Check sheet for the modelled part. Datum: model origin and axes. Units: mm. Face numbers are marked on the shaded views. A direction names the side the tool comes from. Coordinates: 2 decimals unless noted, no trailing zeros. Loops run counter-clockwise (first coordinate to the right, second up) from the corner with the lowest first, then second, coordinate; pieces in that order, holes last.
```python
from build123d import *

# Parameters (mm, degrees)
F1_DEPTH       = 100
F2_W           = 86.5
F2_H           = 50
F3_DEPTH       = 90
F4_W           = 30
F4_H           = 45
F4_W_2         = 14
F4_H_2         = 25
F5_DEPTH       = 60
F7_D           = 4
F7_CSINK_D     = 8.7
F7_CSINK_ANGLE = 90
F8_SIZE        = 2
F9_SIZE        = 3


with BuildPart() as f1:
    # F0 (on Right) → F1 (new body)
    with BuildSketch(Plane.YZ):
        Polygon((-60, 0), (0, 0), (0, 60), (-40, 60), (-40, 100), (-60, 100), align=None)
    extrude(amount=F1_DEPTH)

    # F2 (on face) → F3 (cut)
    with BuildSketch(Plane.XY.offset(100)):
        with Locations((50, -30)):
            Rectangle(F2_W, F2_H)
    extrude(amount=-F3_DEPTH, mode=Mode.SUBTRACT)

    # F4 (on face) → F5 (cut)
    with BuildSketch(Plane(origin=(0, 0, 0), x_dir=(1, 0, 0), z_dir=(0, 0, -1))):
        with Locations((34.25, 22.5)):
            Rectangle(F4_W, F4_H)
        with Locations((74.25, 22.5)):
            Rectangle(F4_W_2, F4_H_2)
    extrude(amount=-F5_DEPTH, mode=Mode.SUBTRACT)

    # F7 (through all)
    with Locations(Plane(origin=(0, -55, 0), x_dir=(-1, 0, 0), z_dir=(0, 1, 0))):
        with Locations((-78.25, 90), (-21.75, 90), (-34.25, 25)):
            CounterSinkHole(F7_D / 2, F7_CSINK_D / 2, counter_sink_angle=F7_CSINK_ANGLE)

    # F8
    f8_edges = [f1.edges().sort_by_distance(p)[0] for p in [
        (74.625, 0, 60),
        (100, 0, 30),
        (0, 0, 30),
        (19.25, 0, 30),
        (49.25, -25, 10),
        (34.25, -45, 10),
        (49.25, 0, 30),
        (100, -20, 60),
        (93.25, -22.5, 60),
        (6.75, -22.5, 60),
        (0, -20, 60),
        (9.625, 0, 60),
        (0, -40, 80),
        (6.75, -40, 80),
        (93.25, -40, 80),
        (100, -40, 80),
        (3.375, -40, 100),
        (0, -50, 100),
        (6.75, -47.5, 100),
        (93.25, -47.5, 100),
        (96.625, -40, 100),
        (100, -50, 100),
        (50, -55, 100),
        (19.25, -2.5, 60),
        (49.25, -2.5, 60),
        (19.25, -25, 10),
    ]]
    chamfer(f8_edges, length=F8_SIZE)

    # F9
    f9_edges = [f1.edges().sort_by_distance(p)[0] for p in [
        (67.25, -22.5, 10),
        (74.25, -10, 10),
        (81.25, -22.5, 10),
        (74.25, -35, 10),
    ]]
    chamfer(f9_edges, length=F9_SIZE)


solid = f1.part
```
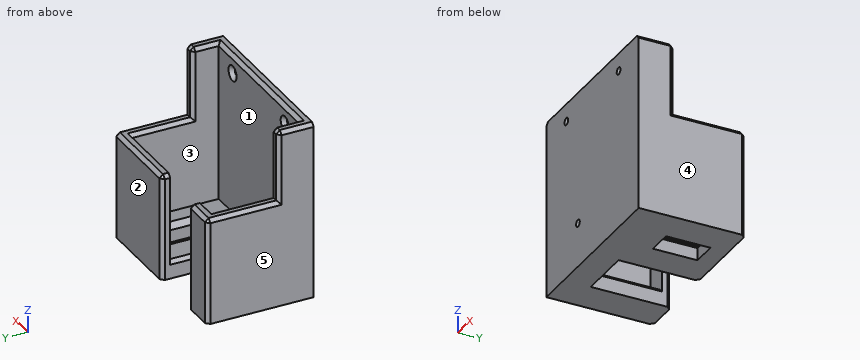
1) Mould release check, pull along X, two halves, no side actions. Record for the marked faces 3, 4 and 5: +X half, -X half, draft (parallel to the pull), parting line (faces both ways), or undercut.
Answer sheet:
face 3: undercut
face 4: +X half
face 5: -X half
2) Scan lines: line 1 (X direction, y = -58.65, z = 90); line 2 (X direction, y = -53.5, z = 77); line 3 (Y direction, x = 51.5, z = 26). Record each from-to range of solid material in increasing order.
Answer sheet:
line 1: x = 0 to 19.75, 23.75 to 76.25, 80.25 to 100
line 2: x = 0 to 6.75, 93.25 to 100
line 3: y = -60 to -55, -5 to 0
3) Section check A-A on x = 34.25. Enter the section's corners in (y, z), plus the area to 3 significant figures.
Answer sheet:
outline: (-60, 0) - (-45, 0) - (-45, 8) - (-47, 10) - (-55, 10) - (-55, 20.65) - (-57.35, 23) - (-60, 23) - close; (-60, 27) - (-57.35, 27) - (-55, 29.35) - (-55, 98) - (-57, 100) - (-60, 100) - close
area: 570 mm2
4) Set-up check for the marked faces 1 and 2: record each of +Z, -Z, +X, -X, +Y, -Y from which the full face is reachable in a straight line by a thin tool's end or side.
Answer sheet:
face 1: +Z
face 2: +Z, -Z, +X, -X, +Y
5) Depth check by flat-ended pin: pin 1 (17 mm diameter, centred on x = 7.5, y = -16, fed in from +Z); pin 2 (0.8 mm diameter, centred on x = 96.5, z = 85.5, fed in from +Y); pin 3 (6.5 mm diameter, centred on x = 32.5, z = 5.5, fed in from +Y). Enter the tip coordinate at first touch or a pass-through.
Answer sheet:
pin 1: stops at z = 60
pin 2: stops at y = -40
pin 3: stops at y = -45
6) Section check D-D on z = 90. Enter the section's corners in (x, y).
Answer sheet:
outline: (0, -60) - (19.75, -60) - (19.75, -57.35) - (17.4, -55) - (6.75, -55) - (6.75, -42) - (4.75, -40) - (2, -40) - (0, -42) - close; (23.75, -60) - (76.25, -60) - (76.25, -57.35) - (73.9, -55) - (26.1, -55) - (23.75, -57.35) - close; (80.25, -60) - (100, -60) - (100, -42) - (98, -40) - (95.25, -40) - (93.25, -42) - (93.25, -55) - (82.6, -55) - (80.25, -57.35) - close
7) Section check B-B on z = 25. Enter the section's corners in (x, y).
Answer sheet:
outline: (0, -60) - (32.25, -60) - (32.25, -57.35) - (29.9, -55) - (6.75, -55) - (6.75, -5) - (19.25, -5) - (19.25, -2) - (17.25, 0) - (2, 0) - (0, -2) - close; (36.25, -60) - (100, -60) - (100, -2) - (98, 0) - (51.25, 0) - (49.25, -2) - (49.25, -5) - (93.25, -5) - (93.25, -55) - (38.6, -55) - (36.25, -57.35) - close
8) Section check C-C on y = -32.5. Enter the section's corners in (x, z), plus the area to 3 significant figures.
Answer sheet:
outline: (0, 0) - (19.25, 0) - (19.25, 8) - (17.25, 10) - (6.75, 10) - (6.75, 58) - (4.75, 60) - (2, 60) - (0, 58) - close; (49.25, 0) - (67.25, 0) - (67.25, 7) - (64.25, 10) - (51.25, 10) - (49.25, 8) - close; (81.25, 0) - (100, 0) - (100, 58) - (98, 60) - (95.25, 60) - (93.25, 58) - (93.25, 10) - (84.25, 10) - (81.25, 7) - close
area: 1,210 mm2
